Check sheet for the modelled part. Datum: model origin and axes. Units: mm. Face numbers are marked on the shaded views. A direction names the side the tool comes from. Coordinates: 2 decimals unless noted, no trailing zeros. Order: outer loops, then holes, each group sorted by start corner. A loop starts at its lowest first (then second) coordinate and runs counter-clockwise, first axis right, second up.
1. Gauge pin test, flat ends, axial feed: pin 1 Ø1.6 at (x, y) = (-1, -8.5) entering from -Z; pin 2 Ø0.6 at (x, y) = (-3, 9) entering from -Z; pin 3 Ø1 at (y, z) = (-8.5, 6.5) entering from -X. Record the tip position at first contact, or that the pin passes through.
2. Draft check along Y on the marked faces 1, 2 and 3. Enter one of: released by +Y, released by -Y, zero draft, split by the parting line, or undercut.
3. Cross-section at C-C (z = 4). Enter the section's corners in (x, y).
4. Cross-section at B-B (x = 1.25). Enter the section's corners in (y, z).
5. Set-up check for the marked faces 4 and 5: record each of +Z, -Z, +X, -X, +Y, -Y from which the full face is reachable in a straight line by a thin tool's end or side.
6. Cross-section at D-D (z = 13.5). Enter the section's corners in (x, y), then the cut area to 3 significant figures.
7. Thickness scan on line 1 (X direction, y = 3.75, z = 36); line 2 (Y direction, x = 7.75, z = 47). Record the ranges inside material, lowest first.
8. Cross-section at A-A (y = 3.75). Enter the section's corners in (x, z).
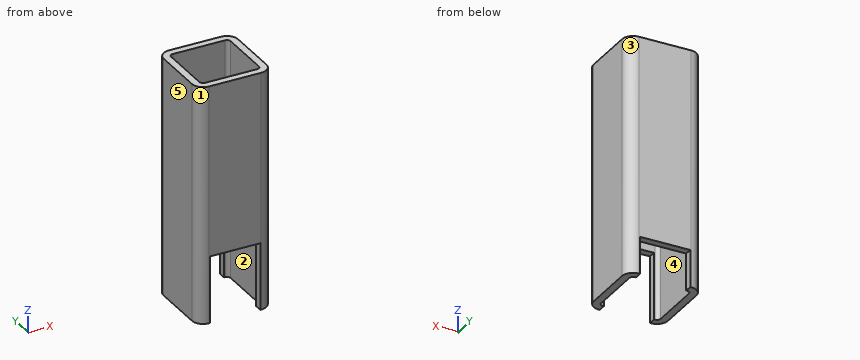
Autodesk Inventor part; units mm, degrees
ref_plane "Start Plane" through (0, 0, 0) normal (0, 0, 1) x (1, 0, 0)
ref_plane "End Plane" through (0, 0, 64) normal (0, 0, 1) x (1, 0, 0)
ref_plane "YZ Plane" through (0, 0, 0) normal (1, 0, 0) x (0, 1, 0)
ref_plane "Start Plane" through (0, 0, 0) normal (0, 0, 1) x (1, 0, 0)
ref_plane "End Plane" through (0, 0, 64) normal (0, 0, 1) x (1, 0, 0)
sketch "Sketch" plane through (0, 0, 0) normal (0, 0, 1) x (1, 0, 0)
  line L0 (-10, -7) -> (-10, 7)
  line L1 (-7, 10) -> (7, 10)
  line L2 (10, 7) -> (10, -7)
  line L3 (7, -10) -> (-7, -10)
  arc A0 (-10, -7) -> (-7, -10) centre (-7, -7) ccw
  arc A1 (-7, 10) -> (-10, 7) centre (-7, 7) ccw
  arc A2 (10, 7) -> (7, 10) centre (7, 7) ccw
  arc A3 (7, -10) -> (10, -7) centre (7, -7) ccw
  arc A4 (-7, 8) -> (-8, 7) centre (-7, 7) ccw
  line L4 (-7, 8) -> (7, 8)
  arc A5 (8, 7) -> (7, 8) centre (7, 7) ccw
  line L5 (8, 7) -> (8, -7)
  arc A6 (7, -8) -> (8, -7) centre (7, -7) ccw
  line L6 (7, -8) -> (-7, -8)
  arc A7 (-8, -7) -> (-7, -8) centre (-7, -7) ccw
  line L7 (-8, -7) -> (-8, 7)
  line L8 (0, 14.8698) -> (0, -14.8698) construction
  line L9 (-14.8698, 0) -> (14.8698, 0) construction
  dimension "d7" = 3
  dimension "d10" = 20
  dimension "d11" = 20
  dimension "d12" = 2
  dimension "d15" = 10
  dimension "d16" = 10
extrude "Body" add sketch "Sketch" along normal up to surface (64 mm away) from surface at 0
sketch "Sketch3" plane through (0, 0, 0) normal (0, 0, 1) x (1, 0, 0)
  line L0 (0, 0) -> (10, 0)
ref_plane "Work Plane3" through (0, 0, 0) normal (0, -1, 0) x (1, 0, 0)
sketch "Sketch4" plane through (0, 0, 0) normal (0, -1, 0) x (1, 0, 0)
  line L0 (-2, 0) -> (12, 0)
  line L1 (-2, 64) -> (12, 64)
  dimension "d18" = 64
sketch "Sketch5" plane through (-7, -10, 0) normal (0, -1, 0) x (1, 0, 0)
  line L0 (14, 64) -> (0, 64)
  line L1 (0, 0) -> (0, 64)
  line L2 (14, 0) -> (0, 0)
  line L3 (14, 18) -> (0, 18)
  line L4 (14, 18) -> (14, 0)
  line L5 (0, 0) -> (0, 64)
  line L6 (0, 0) -> (0, 18)
  line L7 (14, 0) -> (0, 0)
  line L8 (7, 18) -> (7, 15) construction
  line L9 (13.75, 0) -> (0.25, 0)
  line L10 (0.25, 0) -> (0.25, 10)
  line L11 (0.25, 10) -> (13.75, 10)
  line L12 (13.75, 10) -> (13.75, 0)
  line L13 (14, 0) -> (14, 64)
  line L14 (14, 10) -> (0, 10)
  line L15 (0, 10) -> (0, 18)
  line L16 (0, 18) -> (14, 18)
  line L17 (14, 18) -> (14, 10)
  line L18 (13.75, 10) -> (13.75, 18)
  line L19 (0.25, 10) -> (0.25, 18)
  point P0 (7, 0)
  point P1 (7, 0)
  point P2 (0.25, 0)
  point P3 (13.75, 0)
  point P4 (0.25, 18)
  dimension "d19" = 18
  dimension "d23" = 13.5
  dimension "d24" = 10
  dimension "d27" = 8
extrude "Extrusion3" cut sketch "Sketch5" against normal through all contours L12 L2 L10 L11
extrude "Extrusion4" cut sketch "Sketch5" against normal up to next contours L18 L11 L19 L3
equation "\"d7\" = G_IR"
equation "\"d10\" = G_H"
equation "\"d11\" = G_W"
equation "\"d12\" = G_T"
equation "\"d15\" = 0.5 * d10"
equation "\"d16\" = 0.5 * d11"
equation "\"d3\" = G_L"
equation "\"G_W\" = 20"
equation "\"G_H\" = 20"
equation "\"G_T\" = 2"
equation "\"G_IR\" = 3"
equation "\"G_L\" = d18"
equation "\"G_OFFSET_START\" = 0"
equation "\"G_OFFSET_END\" = 0"
equation "\"d14\" = G_OFFSET_END + B_L"
equation "\"B_L\" = 64"
properties part number "ISO 12633-2 - 20x20x2 - 64" material "Steel, Mild"
Data:
1. pin 1: stops at z = 18
1. pin 2: stops at z = 10
1. pin 3: stops at x = -9.83
2. face 1: released by -Y
2. face 2: undercut
2. face 3: released by +Y
3. outline: (-10, -7) arc R3 ccw to (-7, -10) - (-6.75, -10) - (-6.75, -8) - (-7, -8) arc R1 cw to (-8, -7) - (-8, 7) arc R1 cw to (-7, 8) - (-6.75, 8) - (-6.75, 10) - (-7, 10) arc R3 ccw to (-10, 7) - close; (6.75, -10) - (7, -10) arc R3 ccw to (10, -7) - (10, 7) arc R3 ccw to (7, 10) - (6.75, 10) - (6.75, 8) - (7, 8) arc R1 cw to (8, 7) - (8, -7) arc R1 cw to (7, -8) - (6.75, -8) - close
4. outline: (-10, 18) - (-8, 18) - (-8, 64) - (-10, 64) - close; (8, 10) - (10, 10) - (10, 64) - (8, 64) - close
5. face 4: +Z, -Z
5. face 5: +Z, -Z, -X, +Y, -Y
6. outline: (-10, -7) arc R3 ccw to (-7, -10) - (-6.75, -10) - (-6.75, -8) - (-7, -8) arc R1 cw to (-8, -7) - (-8, 7) arc R1 cw to (-7, 8) - (7, 8) arc R1 cw to (8, 7) - (8, -7) arc R1 cw to (7, -8) - (6.75, -8) - (6.75, -10) - (7, -10) arc R3 ccw to (10, -7) - (10, 7) arc R3 ccw to (7, 10) - (-7, 10) arc R3 ccw to (-10, 7) - close
6. area: 110 mm2
7. line 1: x = -10 to -8, 8 to 10
7. line 2: y = -9.9 to -7.66, 7.66 to 9.9
8. outline: (-10, 0) - (-8, 0) - (-8, 64) - (-10, 64) - close; (8, 0) - (10, 0) - (10, 64) - (8, 64) - close
